Autodesk Inventor part; units mm, degrees
ref_plane "Work Plane3" through (0, 0, 250) normal (0, 0, 1) x (1, 0, 0)
ref_plane "Start Plane" through (0, 0, 0) normal (0, 0, 1) x (1, 0, 0)
ref_plane "End Plane" through (0, 0, 400) normal (0, 0, 1) x (1, 0, 0)
sketch "Sketch" plane through (0, 0, 0) normal (0, 0, 1) x (1, 0, 0)
  line L0 (-13, 15) -> (13, 15)
  line L1 (15, 13) -> (15, -13)
  line L2 (-15, 15) -> (15, -15) construction
  line L3 (15, 15) -> (-15, -15) construction
  line L4 (-5.2, 15) -> (-5.2, 14.2)
  line L5 (-5.2, 14.2) -> (-4.1, 14.2)
  line L6 (-4.1, 14.2) -> (-4.1, 12.2)
  line L7 (-4.1, 12.2) -> (-8.25, 12.2)
  line L8 (-8.25, 12.2) -> (-8.25, 10.2)
  line L9 (-8.25, 10.2) -> (-3.85, 5.8)
  line L10 (-3.85, 5.8) -> (3.85, 5.8)
  line L11 (8.25, 12.2) -> (4.1, 12.2)
  line L12 (4.1, 12.2) -> (4.1, 14.2)
  line L13 (4.1, 14.2) -> (5.2, 14.2)
  line L14 (5.2, 14.2) -> (5.2, 15)
  line L15 (8.25, 12.2) -> (8.25, 10.2)
  line L16 (8.25, 10.2) -> (3.85, 5.8)
  line L17 (-2.5, 0) -> (0, 0)
  line L18 (-5.2, -15) -> (-5.2, -14.2)
  line L19 (-5.2, -14.2) -> (-4.1, -14.2)
  line L20 (-4.1, -14.2) -> (-4.1, -12.2)
  line L21 (-4.1, -12.2) -> (-8.25, -12.2)
  line L22 (-8.25, -12.2) -> (-8.25, -10.2)
  line L23 (-8.25, -10.2) -> (-3.85, -5.8)
  line L24 (-3.85, -5.8) -> (3.85, -5.8)
  line L25 (8.25, -12.2) -> (4.1, -12.2)
  line L26 (4.1, -12.2) -> (4.1, -14.2)
  line L27 (4.1, -14.2) -> (5.2, -14.2)
  line L28 (5.2, -14.2) -> (5.2, -15)
  line L29 (8.25, -12.2) -> (8.25, -10.2)
  line L30 (8.25, -10.2) -> (3.85, -5.8)
  line L31 (15, 5.2) -> (14.2, 5.2)
  line L32 (14.2, 5.2) -> (14.2, 4.1)
  line L33 (14.2, 4.1) -> (12.2, 4.1)
  line L34 (12.2, 4.1) -> (12.2, 8.25)
  line L35 (15, -5.2) -> (14.2, -5.2)
  line L36 (14.2, -5.2) -> (14.2, -4.1)
  line L37 (14.2, -4.1) -> (12.2, -4.1)
  line L38 (12.2, -4.1) -> (12.2, -8.25)
  line L39 (12.2, -8.25) -> (10.2, -8.25)
  line L40 (10.2, -8.25) -> (5.8, -3.85)
  line L41 (5.8, -3.85) -> (5.8, 3.85)
  line L42 (5.8, 3.85) -> (10.2, 8.25)
  line L43 (10.2, 8.25) -> (12.2, 8.25)
  line L44 (-15, 5.2) -> (-14.2, 5.2)
  line L45 (-14.2, 5.2) -> (-14.2, 4.1)
  line L46 (-14.2, 4.1) -> (-12.2, 4.1)
  line L47 (-12.2, 4.1) -> (-12.2, 8.25)
  line L48 (-15, -5.2) -> (-14.2, -5.2)
  line L49 (-14.2, -5.2) -> (-14.2, -4.1)
  line L50 (-14.2, -4.1) -> (-12.2, -4.1)
  line L51 (-12.2, -4.1) -> (-12.2, -8.25)
  line L52 (-12.2, -8.25) -> (-10.2, -8.25)
  line L53 (-10.2, -8.25) -> (-5.8, -3.85)
  line L54 (-5.8, -3.85) -> (-5.8, 3.85)
  line L55 (-5.8, 3.85) -> (-10.2, 8.25)
  line L56 (-10.2, 8.25) -> (-12.2, 8.25)
  circle A0 centre (11.5, 11.5) radius 1.65
  circle A1 centre (11.5, -11.5) radius 1.65
  circle A2 centre (-11.5, 11.5) radius 1.65
  circle A3 centre (-11.5, -11.5) radius 1.65
  line L57 (-15, -13) -> (-15, -5.2)
  line L58 (-15, 5.2) -> (-15, 13)
  line L59 (13, -15) -> (5.2, -15)
  line L60 (-5.2, -15) -> (-13, -15)
  arc A4 (-13, 15) -> (-15, 13) centre (-13, 13) ccw
  arc A5 (15, 13) -> (13, 15) centre (13, 13) ccw
  arc A6 (13, -15) -> (15, -13) centre (13, -13) ccw
  arc A7 (-15, -13) -> (-13, -15) centre (-13, -13) ccw
  circle A8 centre (0, 0) radius 2.5
  point P0 (0, 0)
  point P1 (0, 5.8)
  point P2 (0, -2.5)
  point P3 (0, 2.5)
  dimension "d2" = 8.2
  dimension "d3" = 4.1
  dimension "d4" = 10.4
  dimension "d5" = 5.2
  dimension "d8" = 9.2
  dimension "d11" = 16.5
  dimension "d12" = 8.25
  dimension "d14" = 0.8
  dimension "d15" = 2
  dimension "d16" = 2
  dimension "d34" = 0.8
  dimension "d35" = 10.4
  dimension "d36" = 5.2
  dimension "d37" = 8.2
  dimension "d38" = 4.1
  dimension "d39" = 2
  dimension "d40" = 16.5
  dimension "d41" = 8.25
  dimension "d42" = 2
  dimension "d43" = 9.2
  dimension "d44" = 23
  dimension "d45" = 11.5
  dimension "d46" = 23
  dimension "d48" = 3.3
  dimension "d55" = 2
  dimension "d62" = 5
  dimension "d65" = 11.5
  dimension "d66" = 6.4
  dimension "d67" = 3.25
  dimension "d68" = 4.15
  dimension "d69" = 0.8
  dimension "d70" = 2
  dimension "d71" = 2.7577
  dimension "d72" = 5.8
  dimension "d73" = 2.7577
  dimension "d74" = 4.15
  dimension "d75" = 2
  dimension "d76" = 3.25
  dimension "d77" = 2
  dimension "d78" = 1.1
  dimension "d79" = 0.8
  dimension "d80" = 135
  dimension "d81" = 2
  dimension "d82" = 1.1
  dimension "d83" = 7.4
  dimension "d84" = 7.4
  dimension "d85" = 6.4
  dimension "d86" = 6.3
ref_plane "Work Plane3" through (0, 0, 250) normal (0, 0, 1) x (1, 0, 0)
ref_plane "Start Plane" through (0, 0, 0) normal (0, 0, 1) x (1, 0, 0)
ref_plane "End Plane" through (0, 0, 400) normal (0, 0, 1) x (1, 0, 0)
ref_plane "Start Plane1" through (0, 0, 0) normal (0, 0, 1) x (1, 0, 0)
ref_plane "End Plane1" through (0, 0, 400) normal (0, 0, 1) x (1, 0, 0)
ref_plane "Start Plane2" through (0, 0, 15) normal (0, 0, 1) x (1, 0, 0)
ref_plane "End Plane2" through (0, 0, 340) normal (0, 0, 1) x (1, 0, 0)
extrude "Body" add sketch "Sketch" along normal up to surface (325 mm away) from surface at 15 contours L0 L4 L5 L6 L7 L8 L9 L10 L16 L15 L11 L12 L13 L14 A5 L1 L31 L32 L33 L34 L43 L42 L41 L40 L39 L38 L37 L36 L35 A6 L59 L28 L27 L26 L25 L29 L30 L24 L23 L22 L21 L20 L19 L18 L60 A7 L57 L48 L49 L50 L51 L52 L53 L54 L55 L56 L47 L46 L45 L44 L58 A4
sketch "Sketch7" plane through (0, 0, 0) normal (0, 0, 1) x (1, 0, 0)
  line L0 (0, 0) -> (10, 0)
ref_plane "Work Plane10" through (0, 0, 0) normal (0, -1, 0) x (1, 0, 0)
sketch "Sketch8" plane through (0, 0, 0) normal (0, -1, 0) x (1, 0, 0)
  line L0 (-2, 15) -> (12, 15)
  line L1 (-2, 340) -> (12, 340)
  dimension "d100" = 325
ref_plane "Work Plane11" through (-5.2, 225, 15) normal (0, 0, -1) x (-1, 0, 0)
split "Split1" plane through (-5.2, 225, 15) removes the side toward (0, 0, -1)
ref_plane "Work Plane12" through (0, 13, 340) normal (0, 0, 1) x (1, 0, 0)
split "Split2" plane through (0, 13, 340) removes the side toward (0, 0, 1)
equation "\"d38\" = 0.5 * d37"
equation "\"d41\" = 0.5 * d40"
equation "\"d45\" = 0.5 * d44"
equation "\"G_OFFSET_START\" = 0"
equation "\"G_OFFSET_END\" = 0"
equation "\"G_L\" = 500"
equation "\"G_OFFSET_START1\" = 0"
equation "\"G_OFFSET_END1\" = 0"
equation "\"G_OFFSET_START2\" = -15"
equation "\"d95\" = -G_OFFSET_START2"
properties part number "325 mm" material "Aluminum 6061"
The listing builds one solid part. Answer for the finished solid, in the listing's coordinates (mm). A direction names the side the tool comes from. Give positions to 0.01 mm unless a question says otherwise; leave off trailing zeros.
1) Find the intervals of material crossed by L1, parallel to Y at x = 11.5, z = 211.5; L2, parallel to Y at x = 5.5, z = 136.5; L3, parallel to X at y = 6.5, z = 96, in increasing order.
2) For a pull along Y with two mould halves and no side action, classify faces 1 (the face through (15, -9, 175)), 2 (the face through (-9, 15, 175)), 3 (the face through (0, -5.8, 175)), 4 (the face through (5.8, 0, 175)) as pulls with the +Y half, pulls with the -Y half, needs draft (parallel to the pull), parting line crosses it, or undercut.
3) Given P1, Ø0.9, axis at y = -14.5, z = 153, coming from the +X side; P2, Ø0.9, axis at y = 4.5, z = 129, coming from the +X side; P3, Ø8.5, axis at y = 0, z = 153.5, coming from the -X side, each flat-ended and moving along its own axis, determine where each tip first touches the part or whether it passes through.
4) Section A-A (z = 307.5) is taken. Count the separate pieces of the cut face and the enclosed holes in it, and give its area (3 significant figures).
5) A tool of negligible diameter and unlimited length cuts with its end or side. For faces 5 (the face through (0, 5.8, 175)), 6 (the face through (15, 9, 175)), 7 (the face through (-5.8, 0, 175)), from which of +Z, -Z, +X, -X, +Y, -Y can it reach the whole face along a straight path? Write none if from no direction.
Response:
1. L1: y = -15 to -13.15, -9.85 to -8.25, 8.25 to 9.85, 13.15 to 15
1. L2: y = -15 to -12.2, -7.45 to 7.45, 12.2 to 15
1. L3: x = -15 to -12.2, -8.45 to -4.55, 4.55 to 8.45, 12.2 to 15
2. face 1: needs draft
2. face 2: pulls with the +Y half
2. face 3: pulls with the -Y half
2. face 4: undercut
3. P1: stops at x = 14.7
3. P2: stops at x = 14.2
3. P3: stops at x = -14.2
4. separate pieces: 1
4. enclosed holes: 5
4. area: 399 mm2
5. face 5: +Z, -Z, +Y
5. face 6: +Z, -Z, +X, +Y, -Y
5. face 7: +Z, -Z, -X
